For this review, take the finished solid that the model builds, in its own axes (mm). A direction names the side the tool comes from. Give positions to 0.01 mm unless a question says otherwise; leave off trailing zeros. Write each loop counter-clockwise with the first axis right and the second up, starting at its lowest first coordinate (ties: lowest second). Pieces come first, ordered by that corner, then holes. Notation, with made-up numbers: (17, 50) -> (71, 50) arc R29 cw to (71, 82) -> close; hole circle Ø7 at (48.25, -39.75). An arc over 180 degrees is marked (long way). Write item = value, one per line.
```python
from build123d import *

# Parameters (mm, degrees)
F1_R     = 10
F2_R     = 4
F5_DEPTH = 4
F6_DEPTH = 4
F7_R     = 7


with BuildPart() as f3:
    # F1 (on offset) → F3 section 0
    with BuildSketch(Plane.XY.offset(9)):
        Circle(F1_R)
    # F2 (on Top) → F3 section 1
    with BuildSketch(Plane.XY):
        Circle(F2_R)
    loft()

    # F4: F3 across plane


with BuildPart() as f3_1:
    add(f3.part)
    add(f3.part.mirror(Plane.XY))

    # F5 (add): a face of the model
    f5_faces = [f3_1.faces().sort_by_distance(p)[0] for p in [
        (0, 0, -9),
    ]]
    extrude(f5_faces, amount=F5_DEPTH)

    # F6 (add): a face of the model
    f6_faces = [f3_1.faces().sort_by_distance(p)[0] for p in [
        (0, 0, 9),
    ]]
    extrude(f6_faces, amount=F6_DEPTH)

    # F7
    f7_edges = [f3_1.edges().sort_by_distance(p)[0] for p in [
        (-4, 0, 0),
        (-10, 0, -9),
        (-10, 0, 9),
    ]]
    fillet(f7_edges, radius=F7_R)


solid = f3_1.part
```
(1) To check wall thickness, follow probe 1 along Z at (x, y) = (5.5, 7.75); probe 2 along X at (y, z) = (-1.75, -7.5); probe 3 along Z at (x, y) = (7, 3). State the ranges of each line that lie inside material, in increasing order.
Answers below:
probe_1 = -13 to -8.53, 8.53 to 13
probe_2 = -8.82 to 8.82
probe_3 = -13 to -5.42, 5.42 to 13
(2) The part is to be moulded in two halves that separate along Z. For faces 1 (the face through (0, 0, 13)), 2 (the face through (0, 0, -13)), 3 (the face through (-5.315, -4.075, 4.046)), say which applies: released by +Z, released by -Z, zero draft, split by the parting line, or undercut.
Answers below:
face_1 = released by +Z
face_2 = released by -Z
face_3 = undercut
(3) Tool access review of faces 4 (the face through (-1.45, -6.54, -4.05)), 5 (the face through (5.38, 8.43, 12.05)): name each direction out of +Z, -Z, +X, -X, +Y, -Y from which nothing blocks a thin tool from reaching the whole face with its end or side.
Answers below:
face_4 = none
face_5 = +Z, -Z
(4) Take a section at A-A (z = -6.5). Write out the cut boundary in (x, y).
Answers below:
outline = circle Ø16.67 at (0, 0)
(5) For pin 1 (2 mm diameter, centred on x = 0.5, z = 7, fed in from +Y); pin 2 (1 mm diameter, centred on x = 4.5, z = 6, fed in from +Y); pin 3 (4 mm diameter, centred on y = -4, z = 8.5, fed in from +X), all flat-tipped, find the tip position at first contact; note any pin that passes through.
Answers below:
pin_1 = 9.26
pin_2 = 7.12
pin_3 = 9.56
